Autodesk Inventor part; units mm, degrees
ref_plane "YZ Plane" through (0, 0, 0) normal (1, 0, 0) x (0, 1, 0)
ref_plane "XZ Plane" through (0, 0, 0) normal (0, 1, 0) x (-1, 0, 0)
ref_plane "XY Plane" through (0, 0, 0) normal (0, 0, 1) x (1, 0, 0)
sketch "Sketch1" plane through (0, 0, 0) normal (0, 1, 0) x (-1, 0, 0)
  circle A0 centre (-106.68, 0) radius 11
  circle A1 centre (0, 19.05) radius 4.1656
  circle A2 centre (0, -19.05) radius 4.1656
  arc A3 (6.985, 19.05) -> (-0.3988, 26.0236) centre (0, 19.05) ccw
  arc A4 (-0.3988, -26.0236) -> (6.985, -19.05) centre (0, -19.05) ccw
  line L0 (-85.6208, 21.15) -> (-124.655, 21.15)
  line L1 (-124.655, -21.15) -> (-85.6208, -21.15)
  line L2 (-127.83, -17.975) -> (-127.83, 17.975)
  line L3 (6.985, -19.05) -> (6.985, 19.05)
  spline S0 degree 4 poles (-127.83, 17.975) (-127.83, 18.6185) (-127.83, 19.9054) (-126.5854, 21.15) (-125.2985, 21.15) (-124.655, 21.15) knots 0 0 0 0 0 0.5 1 1 1 1 1
  spline S1 degree 4 poles (-127.83, -17.975) (-127.83, -18.6185) (-127.83, -19.9054) (-126.5854, -21.15) (-125.2985, -21.15) (-124.655, -21.15) knots 0 0 0 0 0 0.5 1 1 1 1 1
  line L4 (-85.6208, 21.15) -> (-85.6208, -21.15) construction
  line L5 (-0.3988, 26.0236) -> (-85.6208, 21.15)
  line L6 (-85.6208, -21.15) -> (-0.3988, -26.0236)
  point P0 (0, 0)
  point P1 (-122.18, 15.5)
  point P2 (-91.18, 15.5)
  point P3 (-91.18, -15.5)
  point P4 (-122.18, -15.5)
  dimension "d0" = 106.68
  dimension "d1" = 19.05
  dimension "d2" = 19.05
  dimension "d5" = 22
  dimension "d8" = 8.3312
  dimension "d9" = 8.3312
  dimension "d10" = 13.97
  dimension "d11" = 13.97
  dimension "d52" = 134.815
  dimension "d53" = 42.3
  dimension "d54" = 6.985
  dimension "d55" = 21.15
  dimension "d57" = 98.165
  dimension "d59" = 98.165
  dimension "d61" = 113.665
  dimension "d62" = 129.165
  dimension "d64" = 129.165
  dimension "d66" = 131.64
  dimension "d67" = 131.64
  dimension "d70" = 3.175
  dimension "d71" = 3.175
  dimension "d72" = 5.65
  dimension "d73" = 5.65
  dimension "d74" = 5.65
  dimension "d75" = 5.65
  dimension "d76" = 93.273
  dimension "d77" = 42.3
extrude "Extrusion1" add sketch "Sketch1" along normal blind 3.175
hole "Hole1" at (106.68, 0, 0) at (0, 0, 19.05) at (0, 0, -19.05) at (122.18, 0, 15.5) at (91.18, 0, 15.5) at (91.18, 0, -15.5) at (122.18, 0, -15.5) direction (0, 1, 0) diameter 3.2004 end through all
equation "\"d9\" = d8"
properties part number "x_motor_mount"
The model under review builds one solid part; all positions refer to its coordinate system, in mm. A direction names the side the tool comes from. Give positions to 0.01 mm unless a question says otherwise; leave off trailing zeros. Write each loop counter-clockwise with the first axis right and the second up, starting at its lowest first coordinate (ties: lowest second). Pieces come first, ordered by that corner, then holes.
1. Add section C-C, the plane y = 1.3. Count the separate pieces of the cut face and the enclosed holes in it, plus the area to 3 significant figures.
2. Add section A-A, the plane z = 0. Write out the cut boundary in (x, y) (3 decimals), plus the area to 3 significant figures.
3. Draft analysis for pull direction Z (two halves, no side actions). For faces 1 (the flat face through (127.83, 2, 0)), 2 (the flat face through (105, 2, 21.15)), 3 (the cylindrical face through (120.83, 1.61, -16.36)), state which applies: +Z half, -Z half, draft (parallel to the pull), parting line (faces both ways), or undercut.
4. Add section D-D, the plane z = 7. Write out the cut boundary in (x, y) (3 decimals), plus the area to 3 significant figures.
5. Tool access review of faces 4 (the cylindrical face through (0.54, 1.57, 14.92)), 5 (the flat face through (105, 2, -21.15)): name each direction out of +Z, -Z, +X, -X, +Y, -Y from which nothing blocks a thin tool from reaching the whole face with its end or side.
6. For P1, Ø5, axis at x = 0, z = -19.05, coming from the -Y side, flat-tipped, find the tip position at first contact; note if it passes through.
7. Wall thickness on L1, parallel to Z at x = 122.18, y = 1.2; L2, parallel to Z at x = 106.68, y = 1.75; L3, parallel to X at y = 2.35, z = 15.5 (3 decimals): over which ranges is each line inside the solid? List them lowest first.
8. Add section B-B, the plane x = 122.18. Write out the cut boundary in (y, z) (3 decimals), plus the area to 3 significant figures.
Worked answers:
1. separate pieces: 1
1. enclosed holes: 7
1. area: 5,640 mm2
2. outline: (-6.985, 0) - (95.68, 0) - (95.68, 3.175) - (-6.985, 3.175) - close; (117.68, 0) - (127.83, 0) - (127.83, 3.175) - (117.68, 3.175) - close
2. area: 358 mm2
3. face 1: draft
3. face 2: +Z half
3. face 3: undercut
4. outline: (-6.985, 0) - (98.195, 0) - (98.195, 3.175) - (-6.985, 3.175) - close; (115.165, 0) - (127.83, 0) - (127.83, 3.175) - (115.165, 3.175) - close
4. area: 374 mm2
5. face 4: +Y, -Y
5. face 5: -Z, +X, +Y, -Y
6. P1: passes through
7. L1: z = -21.15 to -17.1, -13.9 to 13.9, 17.1 to 21.15
7. L2: z = -21.15 to -11, 11 to 21.15
7. L3: x = -6.985 to -2.179, 2.179 to 89.58, 92.78 to 120.58, 123.78 to 127.83
8. outline: (0, -21.15) - (3.175, -21.15) - (3.175, -17.1) - (0, -17.1) - close; (0, -13.9) - (3.175, -13.9) - (3.175, 13.9) - (0, 13.9) - close; (0, 17.1) - (3.175, 17.1) - (3.175, 21.15) - (0, 21.15) - close
8. area: 114 mm2
